Geometry: final body of the model. Coordinates: model frame, mm. A direction names the side the tool comes from. Round coordinates to 2 decimals unless told otherwise and drop trailing zeros. Loops run counter-clockwise (first coordinate to the right, second up) from the corner with the lowest first, then second, coordinate; pieces in that order, holes last. Notation, with made-up numbers: (39, -20) - (53, -20) arc R21 ccw to (53, -8) - close; hole circle Ø6 at (40.5, 56.5). An arc over 180 degrees is marked (long way). Return JSON: item names as keys, results as strings. Group by question number.
1. Section B-B on z = 10.75. Return loops of the section in (x, y).
2. Section D-D on z = 2.5. Return loops of the section in (x, y), and give its area (3 significant figures).
3. Section A-A on y = -14.5. Return loops of the section in (x, z).
4. Set-up query: faces 1 (the face through (0, -11.5, 2)), 2 (the face through (-5.556, -6, 15)), 3 (the face through (-6, -15, 22.892)), 4 (the face through (-11, 0, 4)). Return all of +Z, -Z, +X, -X, +Y, -Y with unobstructed straight access to the full face (end or side cutting, diameter ignored); none if empty.
5. First-contact query: pin 1 Ø4 at (x, z) = (5, 2.5) entering from -Y; pin 2 Ø4 at (x, y) = (-3.5, -9.5) entering from +Z; pin 3 Ø10 at (y, z) = (-2, 22.5) entering from -X; pin 4 Ø13.5 at (x, y) = (-1, -4.5) entering from +Z. Flat tips, straight axial feed; report the tip coordinate or a pass-through.
6. Section C-C on y = 0. Return loops of the section in (x, z), and give its area (3 significant figures).
7. Material intervals for probe 1 along Z at (x, y) = (-7, 0); probe 2 along Y at (x, z) = (-10, 4.75); probe 3 along Z at (x, y) = (-0.75, 5.25), sorted ascending.
8. Draft query along X for faces 5 (the face through (-6.664, -13.452, 15.397)), 6 (the face through (0, 0, 0)), 7 (the face through (11.5, 0, 2)). Return one class per face: +X half, -X half, draft (parallel to the pull), parting line (faces both ways), or undercut.
from build123d import *

# Parameters (mm, degrees)
F0_W         = 23
F0_H         = 23
F1_DEPTH     = 4
F2_W         = 4.5
F2_H         = 23
F3_DEPTH     = 23
F4_W         = 4.5
F4_H         = 14.783909363
F5_DEPTH     = 6
F7_D         = 11
F9_D         = 3.1
F10_T1_DEPTH = 39.5
F10_T3_DEPTH = 36.3734207923


# Not quite as in the source:
# - a fillet or chamfer that OpenCascade refuses, or shapes differently, is made with other operations: its cross-section is extruded or revolved along the edge and cut away or added


with BuildPart() as f1:
    # F0 (on Top) → F1 (new body)
    with BuildSketch(Plane.XY):
        Rectangle(F0_W, F0_H)
    extrude(amount=F1_DEPTH)

    # F2 (on face) → F3 (join)
    with BuildSketch(Plane.XY.offset(4)):
        with Locations((-7.8062060252, 0)):
            Rectangle(F2_W, F2_H)
    extrude(amount=F3_DEPTH)

    # F4 (on face) → F5 (join)
    with BuildSketch(Plane.XZ.offset(11.5)):
        with Locations((-7.8062060252, 15.5)):
            Rectangle(F4_W, F4_H)
    extrude(amount=F5_DEPTH)

    # F7 (through all)
    with Locations(Plane(origin=(-10.0562060252, 0, 0), x_dir=(0, -1, 0), z_dir=(-1, 0, 0))):
        with Locations((0, 15.7216731459)):
            Hole(F7_D / 2)

    # F9 (through all)
    with Locations(Plane.XY.offset(22.8919546815)):
        with Locations((-7.8062060252, -14.5)):
            Hole(F9_D / 2)

    # F10: fillet of radius 7 on 2 edges, made by hand

    # F10_s2 → F10_t1 (cut)
    with BuildSketch(Plane.YZ.offset(-27.5562060252)):
        with BuildLine():
            ThreePointArc((11.5, 20), (9.4497474683, 24.9497474683), (4.5, 27))
            Line((4.5, 27), (11.5, 27))
            Line((11.5, 27), (11.5, 20))
        make_face()
    extrude(amount=F10_T1_DEPTH, mode=Mode.SUBTRACT)

    # F10_s4 → F10_t3 (cut)
    with BuildSketch(Plane.YZ.offset(-25.9929164214)):
        with BuildLine():
            ThreePointArc((-5.1253158415, 27), (-8.9171700865, 25.8840327485), (-11.5, 22.8919546815))
            Line((-11.5, 22.8919546815), (-11.5, 27))
            Line((-11.5, 27), (-5.1253158415, 27))
        make_face()
    extrude(amount=F10_T3_DEPTH, mode=Mode.SUBTRACT)


solid = f1.part
Taken from the geometry:
{
 "1": {"outline": "(-10.06, -17.5) - (-5.56, -17.5) - (-5.56, -2.35) - (-10.06, -2.35) - close; (-10.06, 2.35) - (-5.56, 2.35) - (-5.56, 11.5) - (-10.06, 11.5) - close; hole circle Ø3.1 at (-7.81, -14.5)"},
 "2": {"outline": "(-11.5, -11.5) - (11.5, -11.5) - (11.5, 11.5) - (-11.5, 11.5) - close", "area": "529 mm2"},
 "3": {"outline": "(-10.06, 8.11) - (-9.36, 8.11) - (-9.36, 22.89) - (-10.06, 22.89) - close; (-6.26, 8.11) - (-5.56, 8.11) - (-5.56, 22.89) - (-6.26, 22.89) - close"},
 "4": {"face 1": "-Z, +X, -X, -Y", "face 2": "+Z, +X, +Y, -Y", "face 3": "+Z, +X, -X, -Y", "face 4": "+Z, -X, +Y, -Y"},
 "5": {"pin 1": "y = -11.5", "pin 2": "z = 4", "pin 3": "x = -10.06", "pin 4": "z = 27"},
 "6": {"outline": "(-11.5, 0) - (11.5, 0) - (11.5, 4) - (-5.56, 4) - (-5.56, 10.22) - (-10.06, 10.22) - (-10.06, 4) - (-11.5, 4) - close; (-10.06, 21.22) - (-5.56, 21.22) - (-5.56, 27) - (-10.06, 27) - close", "area": "146 mm2"},
 "7": {"probe 1": "0 to 10.22, 21.22 to 27", "probe 2": "-11.5 to 11.5", "probe 3": "0 to 4"},
 "8": {"face 5": "undercut", "face 6": "draft", "face 7": "+X half"}
}
